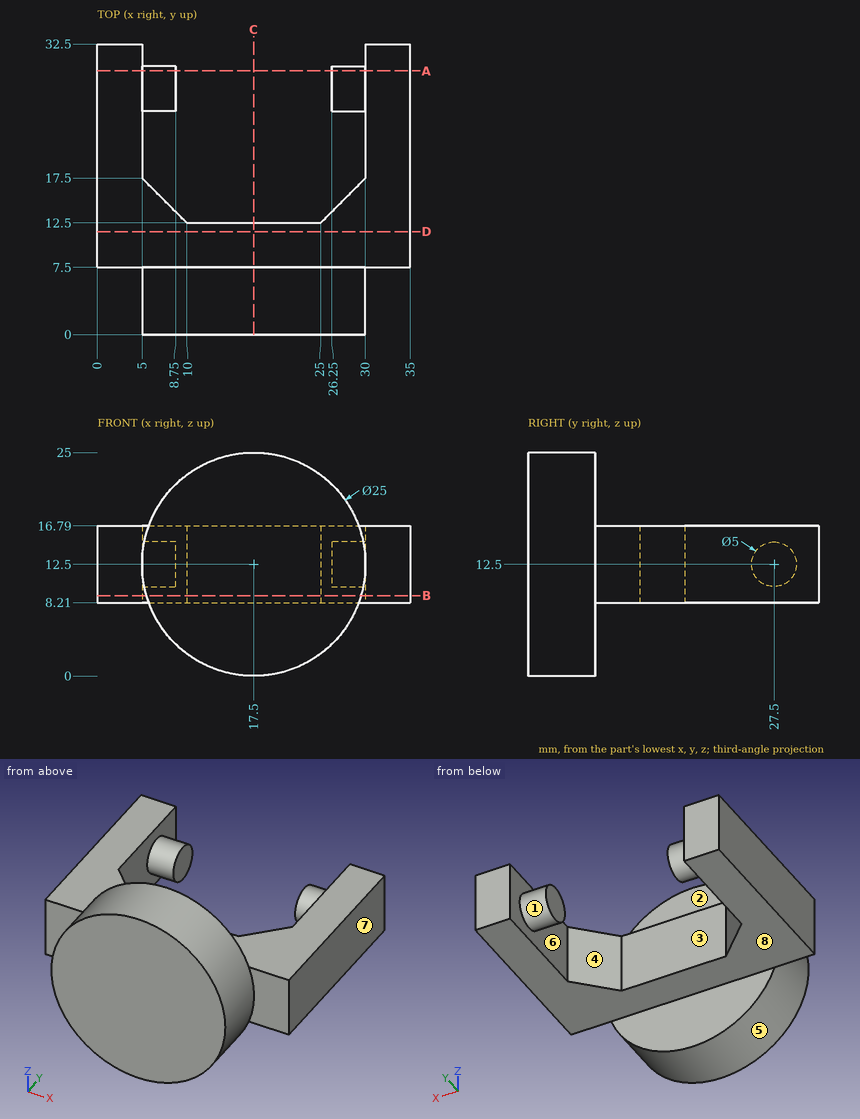
The figure shows three views and two pictorial views of one solid part (mm, origin at its lowest corner). Answer the questions. A direction names the side the tool comes from. Round coordinates to 2 decimals unless told otherwise and drop trailing zeros. Write each loop counter-clockwise with the first axis right and the second up, starting at its lowest first coordinate (ties: lowest second). Pieces come first, ordered by that corner, then holes. Notation, with made-up numbers: (51, 57) -> (85, 57) arc R15 cw to (85, 75) -> close; hole circle Ø1 at (55, 49). An arc over 180 degrees is marked (long way). Answer as a JSON object with one key per item and string values. Group by question number.
Q1. Determine the mould class of the marked faces 5, 6, 7 and 8 for opening direction X: pulls with the +X half, pulls with the -X half, needs draft (parallel to the pull), parting line crosses it, or undercut.
Q2. Section C-C (x = 17.5) is taken. Write down the section's boundary in (y, z), plus the area to 3 significant figures.
Q3. Section A-A (y = 29.5) is taken. Write down the section's boundary in (x, z).
Q4. Each of these flat-tipped pins is pushed along its axis until it touches: pin 1 Ø12.5 at (x, y) = (22, 22.5) entering from -Z (1 decimal); pin 2 Ø9 at (x, z) = (17.5, 4) entering from +Y; pin 3 Ø6.5 at (x, z) = (19, 22) entering from +Y. Where does it stop, or does it pass through?
Q5. Straight lines are drawn through the part: line 1 along X through (y, z) = (31.5, 13.5); line 2 along Y through (x, z) = (3, 12); line 3 along Z through (x, y) = (17, 2). For each, find the intervals that lie inside material, in ascending order.
Q6. Section B-B (z = 9) is taken. Write down the section's boundary in (x, y), plus the area to 3 significant figures.
Q7. Section D-D (y = 11.5) is taken. Write down the section's boundary in (x, z), plus the area to 3 significant figures.
Q8. Which of the six approach directions +Z, -Z, +X, -X, +Y, -Y give full straight-line access (tool end or side, diameter ignored) to the marked faces 1, 2, 3 and 4?
Check values:
{
 "1": {"face 5": "parting line crosses it", "face 6": "undercut", "face 7": "pulls with the +X half", "face 8": "needs draft"},
 "2": {"outline": "(0, 0) -> (7.5, 0) -> (7.5, 8.21) -> (12.5, 8.21) -> (12.5, 16.79) -> (7.5, 16.79) -> (7.5, 25) -> (0, 25) -> close", "area": "230 mm^2"},
 "3": {"outline": "(0, 8.21) -> (5, 8.21) -> (5, 11) -> (8.75, 11) -> (8.75, 14) -> (5, 14) -> (5, 16.79) -> (0, 16.79) -> close; (26.25, 11) -> (30, 11) -> (30, 8.21) -> (35, 8.21) -> (35, 16.79) -> (30, 16.79) -> (30, 14) -> (26.25, 14) -> close"},
 "4": {"pin 1": "z = 10", "pin 2": "y = 12.5", "pin 3": "y = 7.5"},
 "5": {"line 1": "0 to 5, 30 to 35", "line 2": "7.5 to 32.5", "line 3": "0.01 to 24.99"},
 "6": {"outline": "(0, 7.5) -> (5.5, 7.5) -> (5.5, 0) -> (29.5, 0) -> (29.5, 7.5) -> (35, 7.5) -> (35, 32.5) -> (30, 32.5) -> (30, 17.5) -> (25, 12.5) -> (10, 12.5) -> (5, 17.5) -> (5, 32.5) -> (0, 32.5) -> close", "area": "580 mm^2"},
 "7": {"outline": "(0, 8.21) -> (35, 8.21) -> (35, 16.79) -> (0, 16.79) -> close", "area": "300 mm^2"},
 "8": {"face 1": "none", "face 2": "+Z, +X, -X, +Y", "face 3": "+Z, -Z, +Y", "face 4": "+Z, -Z"}
}
